from build123d import *

# Parameters (mm, degrees)
F1_DEPTH = 19.05
F2_R     = 6.35
F3_R     = 6.35


with BuildPart() as f1:
    # F0 (on Right) → F1 (new body)
    with BuildSketch(Plane.YZ):
        with BuildLine():
            Line((0, 133.35), (0, 0))
            Line((0, 0), (50.8, 0))
            Line((50.8, 0), (50.8, 6.35))
            ThreePointArc((50.8, 6.35), (58.239488, 24.310512), (76.2, 31.75))
            Line((76.2, 31.75), (241.3, 31.75))
            ThreePointArc((241.3, 31.75), (259.260512, 24.310512), (266.7, 6.35))
            Line((266.7, 6.35), (266.7, 0))
            Line((266.7, 0), (317.5, 0))
            Line((317.5, 0), (317.5, 266.7))
            Line((317.5, 266.7), (158.75, 266.7))
            Line((158.75, 266.7), (158.75, 133.35))
            Line((158.75, 133.35), (0, 133.35))
        make_face()
    extrude(amount=F1_DEPTH)

    # F2
    f2_edges = [f1.edges().sort_by_distance(p)[0] for p in [
        (19.05, 158.75, 31.75),
    ]]
    fillet(f2_edges, radius=F2_R)

    # F3
    f3_edges = [f1.edges().sort_by_distance(p)[0] for p in [
        (0, 158.75, 31.75),
    ]]
    fillet(f3_edges, radius=F3_R)


solid = f1.part
For this review, take the finished solid that the model builds, in its own axes (mm). A direction names the side the tool comes from. Round coordinates to 2 decimals unless told otherwise and drop trailing zeros. Loops run counter-clockwise (first coordinate to the right, second up) from the corner with the lowest first, then second, coordinate; pieces in that order, holes last. Notation, with made-up numbers: (35, 29.5) - (65, 29.5) arc R14 cw to (65, 51.5) - close; hole circle Ø10 at (82.25, -5.5). An arc over 180 degrees is marked (long way). Put each result on its own line as item: value. Start each with the question number.
1. Consider section C-C on x = 3. State the section outline as (y, z) points.
2. Insertion check: P1, Ø1.9, axis at x = 9, y = 134.5, coming from the -Z side; P2, Ø8, axis at x = 13, z = 204, coming from the -Y side; P3, Ø2, axis at x = 8.5, y = 73.5, coming from the +Z side. Each pin has a flat end and moves straight along its axis. Give the tip position at first contact, or say it passes through.
3. For faces 1 (the cylindrical face through (17.14, 48.99, 3.22)), 2 (the flat face through (9, 80, 133.35)), 3 (the flat face through (9, 266.7, 3)), list the 3-axis set-ups (+Z, -Z, +X, -X, +Y, -Y) from which the entire face can be reached by the end or side of a thin tool; tool diameter is ignored.
4. Mouldability with a two-part tool opening along Y and no side actions: class faces 4 (the flat face through (9, 317.5, 131)), 5 (the flat face through (0, 192, 135)), 6 (the flat face through (9, 0, 68)), 7 (the flat face through (9, 50.8, 3)) as +Y half, -Y half, draft (parallel to the pull), parting line (faces both ways), or undercut.
5. For probe 1 along Z at (x, y) = (12.25, 113); probe 2 along Y at (x, z) = (15, 139); probe 3 along Y at (x, z) = (17.25, 20), list the stretches that pass through material, from the lowest coordinate up. Write a range as [from, to].
6. Consider section B-B on z = 192. State the section outline as (x, y) points, plus the area to 3 significant figures.
7. Consider section A-A on y = 101.5. State the section outline as (x, z) points, plus the area to 3 significant figures.
8. Consider section D-D on y = 189. State the section outline as (x, z) points, plus the area to 3 significant figures.
Result sheet:
1. outline: (0, 0) - (49.84, 0) - (49.84, 6.35) arc R26.36 cw to (76.2, 32.71) - (241.3, 32.71) arc R26.36 cw to (267.66, 6.35) - (267.66, 0) - (317.5, 0) - (317.5, 266.7) - (158.75, 266.7) - (158.75, 133.35) - (0, 133.35) - close
2. P1: z = 31.75
2. P2: y = 158.75
2. P3: z = 133.35
3. face 1: -Z, +X
3. face 2: +Z, +X, -X, -Y
3. face 3: -Z, +X, -X
4. face 4: +Y half
4. face 5: draft
4. face 6: -Y half
4. face 7: undercut
5. probe 1: [31.75, 133.35]
5. probe 2: [158.75, 317.5]
5. probe 3: [0, 52.53], [264.97, 317.5]
6. outline: (0, 158.75) - (19.05, 158.75) - (19.05, 317.5) - (0, 317.5) - close
6. area: 3,020 mm^2
7. outline: (0, 38.1) arc R6.35 ccw to (6.35, 31.75) - (12.7, 31.75) arc R6.35 ccw to (19.05, 38.1) - (19.05, 133.35) - (0, 133.35) - close
7. area: 1,920 mm^2
8. outline: (0, 38.1) arc R6.35 ccw to (6.35, 31.75) - (12.7, 31.75) arc R6.35 ccw to (19.05, 38.1) - (19.05, 266.7) - (0, 266.7) - close
8. area: 4,460 mm^2
